Check sheet for the modelled part. Datum: model origin and axes. Units: mm. Face numbers are marked on the shaded views. A direction names the side the tool comes from. Coordinates: 2 decimals unless noted, no trailing zeros. Loops run counter-clockwise (first coordinate to the right, second up) from the corner with the lowest first, then second, coordinate; pieces in that order, holes last. Notation, with made-up numbers: (11.25, -18.5) - (48.25, -18.5) arc R18 cw to (48.25, -3.5) - close; hole circle Ø11 at (5.5, -22). An arc over 180 degrees is marked (long way). Write each question's results on one line, items separated by ' | '. Start each with the question number.
1. Cross-section at D-D (y = 2.25). Record the cut outline in (x, z), and give its area (3 significant figures).
2. Cross-section at C-C (z = 11.75). Record the cut outline in (x, y), and give its area (3 significant figures).
3. Cross-section at B-B (x = 0). Record the cut outline in (y, z).
4. Draft check along Y on the marked faces 4, 5 and 6. Enter one of: released by +Y, released by -Y, zero draft, split by the parting line, or undercut.
5. Tool access check on the marked faces 1, 2 and 3. Record the directions out of +Z, -Z, +X, -X, +Y, -Y that give a thin tool (end or side, any length) a straight path to the whole face; none if there is none.
6. Gauge pin test, flat ends, axial feed: P1, Ø2.5, axis at x = 0.5, z = 10, coming from the +Y side; P2, Ø1.5, axis at y = -4, z = 11.5, coming from the +X side; P3, Ø3, axis at x = 3, z = 2.5, coming from the +Y side; P4, Ø1, axis at x = -2, z = 2, coming from the -Y side. Record the tip position at first contact, or that the pin passes through.
7. Thickness scan on line 1 (Y direction, x = 0, z = 6.8); line 2 (X direction, y = 2.75, z = 3.75); line 3 (X direction, y = -2.5, z = 8.5). Record the ranges inside material, lowest first. Write a range as [from, to].
8. Cross-section at A-A (y = 0). Record the cut outline in (x, z).
```python
from build123d import *

# Parameters (mm, degrees)
SKETCH032_R     = 5.5
PAD020_DEPTH    = 6
SKETCH033_R     = 5.5
PAD021_DEPTH    = 1
SKETCH034_R     = 1.9
POCKET010_DEPTH = 5
SKETCH035_R     = 5.5
PAD022_DEPTH    = 8


with BuildPart() as part:
    # Sketch032 → Pad020 (new body)
    with BuildSketch(Plane.XY):
        Circle(SKETCH032_R)
        with BuildLine():
            Line((-2.3, 1.926136), (-2.3, -1.926136))
            ThreePointArc((-2.3, -1.926136), (0, -3), (2.3, -1.926136))
            Line((2.3, 1.926136), (2.3, -1.926136))
            ThreePointArc((2.3, 1.926136), (0, 3), (-2.3, 1.926136))
        make_face(mode=Mode.SUBTRACT)
    extrude(amount=PAD020_DEPTH)

    # Sketch033 (on Face7 of Pad020) → Pad021 (join)
    with BuildSketch(Plane.XY.offset(6)):
        Circle(SKETCH033_R)
    extrude(amount=PAD021_DEPTH)

    # Sketch034 (on Face1 of Pad021) → Pocket010 (cut)
    with BuildSketch(Plane.XY.offset(7)):
        Circle(SKETCH034_R)
    extrude(amount=-POCKET010_DEPTH, mode=Mode.SUBTRACT)

    # Sketch035 (on Face1 of Pocket010) → Pad022 (join)
    with BuildSketch(Plane.XY.offset(7)):
        Circle(SKETCH035_R)
        Polygon((-3.66998, -1.59099), (-3.66998, 1.59099), (-1.59099, 1.59099), (-1.59099, 3.66998), (1.59099, 3.66998), (1.59099, 1.59099), (3.66998, 1.59099), (3.66998, -1.59099), (1.59099, -1.59099), (1.59099, -3.66998), (-1.59099, -3.66998), (-1.59099, -1.59099), align=None, mode=Mode.SUBTRACT)
    extrude(amount=PAD022_DEPTH)


solid = part.part
```
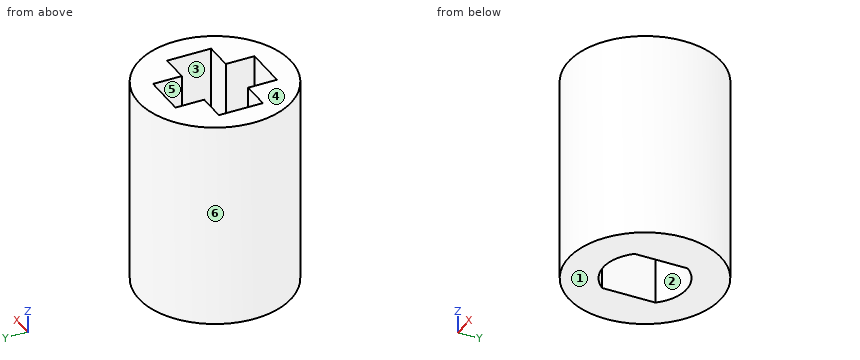
Established:
1) outline: (-5.02, 0) - (-1.98, 0) - (-1.98, 6) - (1.98, 6) - (1.98, 0) - (5.02, 0) - (5.02, 15) - (1.59, 15) - (1.59, 7) - (-1.59, 7) - (-1.59, 15) - (-5.02, 15) - close | area: 101 mm^2
2) outline: circle Ø11 at (0, 0); hole (-3.67, -1.59) - (-1.59, -1.59) - (-1.59, -3.67) - (1.59, -3.67) - (1.59, -1.59) - (3.67, -1.59) - (3.67, 1.59) - (1.59, 1.59) - (1.59, 3.67) - (-1.59, 3.67) - (-1.59, 1.59) - (-3.67, 1.59) - close | area: 58.4 mm^2
3) outline: (-5.5, 0) - (-3, 0) - (-3, 6) - (-1.9, 6) - (-1.9, 7) - (-3.67, 7) - (-3.67, 15) - (-5.5, 15) - close; (1.9, 6) - (3, 6) - (3, 0) - (5.5, 0) - (5.5, 15) - (3.67, 15) - (3.67, 7) - (1.9, 7) - close
4) face 4: zero draft | face 5: undercut | face 6: split by the parting line
5) face 1: -Z, +X, -X, +Y, -Y | face 2: -Z | face 3: +Z
6) P1: y = 5.5 | P2: x = 4.44 | P3: y = 5.29 | P4: y = -5.29
7) line 1: [-5.5, -1.9], [1.9, 5.5] | line 2: [-4.76, -1.2], [1.2, 4.76] | line 3: [-4.9, -1.59], [1.59, 4.9]
8) outline: (-5.5, 0) - (-2.3, 0) - (-2.3, 6) - (-1.9, 6) - (-1.9, 7) - (-3.67, 7) - (-3.67, 15) - (-5.5, 15) - close; (1.9, 6) - (2.3, 6) - (2.3, 0) - (5.5, 0) - (5.5, 15) - (3.67, 15) - (3.67, 7) - (1.9, 7) - close
